```python
from build123d import *

# Parameters (mm, degrees)
F0_W     = 33.077959
F0_H     = 62.316516
F1_DEPTH = 25.4
F4_D     = 5.1054
F5_D     = 5.1054


with BuildPart() as f1:
    # F0 (on Top) → F1 (new body)
    with BuildSketch(Plane.XY):
        with Locations((-10.229463, -11.399078)):
            Rectangle(F0_W, F0_H)
    extrude(amount=F1_DEPTH)

    # F4 (through all)
    with Locations(Plane.YZ.offset(6.309517)):
        with Locations((-29.974079, 14.525045), (-4.574079, 14.525045)):
            Hole(F4_D / 2)

    # F5 (through all)
    with Locations(Plane.XY.offset(25.4)):
        with Locations((-14.157081, 9.891412), (-14.157081, -15.508588)):
            Hole(F5_D / 2)


solid = f1.part
```
Input: part model. Units: mm. Frame: model coordinates. Give positions to 0.01 mm unless a question says otherwise; leave off trailing zeros. Write each loop counter-clockwise with the first axis right and the second up, starting at its lowest first coordinate (ties: lowest second). Pieces come first, ordered by that corner, then holes. Notation, with made-up numbers: (24, 68) - (43, 68) arc R16 ccw to (43, 88) - close; hole circle Ø5 at (-22.75, 60). An arc over 180 degrees is marked (long way). Write item = value, one per line. Start each with the question number.
1) Draft query along X for faces 1 (the face through (-10, -11, 0)), 2 (the face through (-16.515, -16.486, 12.522)), 3 (the face through (-26.768, -12, 13)). Return one class per face: pulls with the +X half, pulls with the -X half, needs draft (parallel to the pull), parting line crosses it, or undercut.
2) Cut plane C-C (z = 17.75). Return loops of the section in (x, y), and give its area (3 significant figures).
3) Material intervals for L1, parallel to Y at x = -14, z = 11.25; L2, parallel to Y at x = -18.5, z = 15; L3, parallel to X at y = -16, z = 2.75, sorted ascending. Write a range as [from, to].
4) Cut plane D-D (y = -30). Return loops of the section in (x, z), and give its area (3 significant figures).
5) Cut plane B-B (y = -5.5). Return loops of the section in (x, z).
6) Cut plane A-A (x = -13.5). Return loops of the section in (y, z), and give its area (3 significant figures).
Answers follow:
q1.face_1 = needs draft
q1.face_2 = undercut
q1.face_3 = pulls with the -X half
q2.outline = (-26.77, -42.56) - (6.31, -42.56) - (6.31, 19.76) - (-26.77, 19.76) - close; hole circle Ø5.11 at (-14.16, -15.51); hole circle Ø5.11 at (-14.16, 9.89)
q2.area = 2,020 mm^2
q3.L1 = [-42.56, -18.06], [-12.96, 7.34], [12.44, 19.76]
q3.L2 = [-42.56, -32.48], [-27.47, -7.08], [-2.07, 19.76]
q3.L3 = [-26.77, -16.66], [-11.65, 6.31]
q4.outline = (-26.77, 0) - (6.31, 0) - (6.31, 11.97) - (-26.77, 11.97) - close; (-26.77, 17.08) - (6.31, 17.08) - (6.31, 25.4) - (-26.77, 25.4) - close
q4.area = 671 mm^2
q5.outline = (-26.77, 0) - (6.31, 0) - (6.31, 12.15) - (-26.77, 12.15) - close; (-26.77, 16.9) - (6.31, 16.9) - (6.31, 25.4) - (-26.77, 25.4) - close
q6.outline = (-42.56, 0) - (-17.98, 0) - (-17.98, 25.4) - (-42.56, 25.4) - close; (-13.04, 0) - (7.42, 0) - (7.42, 25.4) - (-13.04, 25.4) - close; (12.36, 0) - (19.76, 0) - (19.76, 25.4) - (12.36, 25.4) - close; hole circle Ø5.11 at (-29.97, 14.53); hole circle Ø5.11 at (-4.57, 14.53)
q6.area = 1,290 mm^2
